from build123d import *

# Parameters (mm, degrees)
SKETCH1_R               = 1.5
BOSS_EXTRUDE1_DEPTH     = 23
SKETCH2_W               = 13
SKETCH2_H               = 23.129290295
CUT_EXTRUDE1_DEPTH      = 16
CUT_EXTRUDE1_DEPTH_BACK = 16
FILLET1_R               = 3
SKETCH3_R               = 1.5
CUT_EXTRUDE2_DEPTH      = 6


with BuildPart() as part:
    # Sketch1 → Boss-Extrude1 (new body)
    with BuildSketch(Plane.XY):
        with BuildLine():
            Line((-15, 0), (15, 0))
            Line((15, 0), (8.141386903, 22.862043657))
            ThreePointArc((8.141386903, 22.862043657), (7.058699636, 24.406878785), (5.267908047, 25))
            Line((5.267908047, 25), (-5.267908047, 25))
            ThreePointArc((-5.267908047, 25), (-7.058699636, 24.406878785), (-8.141386903, 22.862043657))
            Line((-8.141386903, 22.862043657), (-15, 0))
        make_face()
        with Locations((0, 15)):
            Circle(SKETCH1_R, mode=Mode.SUBTRACT)
    extrude(amount=BOSS_EXTRUDE1_DEPTH)

    # Sketch2 → Cut-Extrude1 (cut, two sides)
    with BuildSketch(Plane(origin=(0, 0, 0), x_dir=(0, 0, -1), z_dir=(1, 0, 0))) as cut_extrude1_sk:
        with Locations((-11.5, 16.564645148)):
            Rectangle(SKETCH2_W, SKETCH2_H)
    extrude(amount=CUT_EXTRUDE1_DEPTH, mode=Mode.SUBTRACT)
    extrude(cut_extrude1_sk.sketch, amount=-CUT_EXTRUDE1_DEPTH_BACK, mode=Mode.SUBTRACT)

    # Fillet1
    fillet1_edges = [part.edges().sort_by_distance(p)[0] for p in [
        (0, 5, 5),
        (0, 5, 18),
    ]]
    fillet(fillet1_edges, radius=FILLET1_R)

    # Sketch3 → Cut-Extrude2 (cut, through all)
    with BuildSketch(Plane(origin=(0, 5, 0), x_dir=(1, 0, 0), z_dir=(0, 1, 0))):
        with Locations((0, -11.5)):
            Circle(SKETCH3_R)
    extrude(amount=-CUT_EXTRUDE2_DEPTH, mode=Mode.SUBTRACT)


solid = part.part
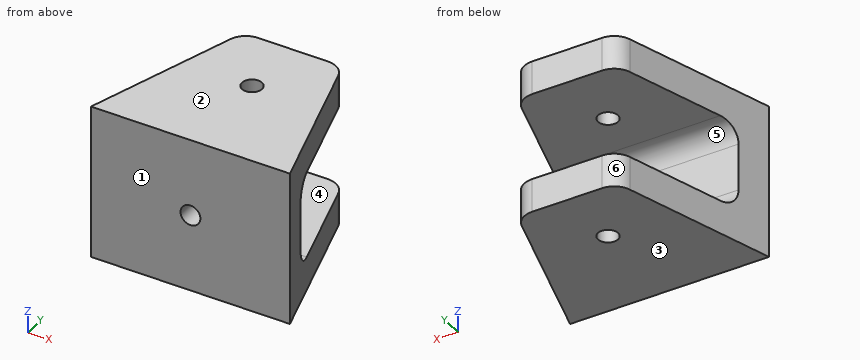
Input: part model. Units: mm. Frame: model coordinates. Face numbers are marked on the shaded views. A direction names the side the tool comes from. Coordinates: 2 decimals unless noted, no trailing zeros. Order: outer loops, then holes, each group sorted by start corner. A loop starts at its lowest first (then second) coordinate and runs counter-clockwise, first axis right, second up. Notation, with made-up numbers: M -20.75,43 L -4.75,43 A18 ccw -4.75,73 Z; hole C 26,63.25 d2. An arc over 180 degrees is marked long. Answer as CSV lines item,"result".
1. Section D-D (y = 15). Return the cut outline in (x, z).
Reported:
outline,"M -10.5,0 L -1.5,0 L -1.5,5 L -10.5,5 Z; M -10.5,18 L -1.5,18 L -1.5,23 L -10.5,23 Z; M 1.5,0 L 10.5,0 L 10.5,5 L 1.5,5 Z; M 1.5,18 L 10.5,18 L 10.5,23 L 1.5,23 Z"
2. Section A-A (y = 9.5). Return the cut outline in (x, z).
Reported:
outline,"M -12.15,0 L 12.15,0 L 12.15,5 L -12.15,5 Z; M -12.15,18 L 12.15,18 L 12.15,23 L -12.15,23 Z"
3. Pull-direction query (Z, two-part tool) for the marked faces 1, 2, 3 and 4; classes: released by +Z, released by -Z, zero draft, split by the parting line, or undercut.
Reported:
face 1,"zero draft"
face 2,"released by +Z"
face 3,"released by -Z"
face 4,"undercut"
4. Section B-B (z = 11.5). Return the cut outline in (x, y).
Reported:
outline,"M -15,0 L -1.5,0 L -1.5,5 L -13.5,5 Z; M 1.5,0 L 15,0 L 13.5,5 L 1.5,5 Z"
5. First-contact query: P1, Ø5.5, axis at x = -4.5, z = 12.5, coming from the +Y side; P2, Ø1.5, axis at y = 4, z = 12.5, coming from the -X side (3 decimals); P3, Ø1, axis at y = 12, z = 4.5, coming from the -X side. Flat tips, straight axial feed; report the tip coordinate or a pass-through.
Reported:
P1,"y = 5.01"
P2,"x = -14.025"
P3,"x = -11.55"
6. Material intervals for line 1 (Z direction, x = 3.5, y = 9.25); line 2 (Z direction, x = 0, y = 2.5); line 3 (Y direction, x = 0, z = 19.9), sorted ascending. Write a range as from..to.
Reported:
line 1,"0..5, 18..23"
line 2,"0..10, 13..23"
line 3,"0..13.5, 16.5..25"
7. Access query for the marked faces 5 and 6. Directions: +Z, -Z, +X, -X, +Y, -Y. A direction counts if a zero-diameter tool reaches every point of the face in a straight line with its end or side. Return the directions, or none.
Reported:
face 5,"+X, -X, +Y"
face 6,"+Z, -Z, -X, +Y"
8. Section C-C (x = 0). Return the cut outline in (y, z).
Reported:
outline,"M 0,0 L 13.5,0 L 13.5,5 L 8,5 A3 cw 5,8 L 5,10 L 0,10 Z; M 0,13 L 5,13 L 5,15 A3 cw 8,18 L 13.5,18 L 13.5,23 L 0,23 Z; M 16.5,0 L 25,0 L 25,5 L 16.5,5 Z; M 16.5,18 L 25,18 L 25,23 L 16.5,23 Z"
